Geometry: final body of the model. Coordinates: model frame, mm. A direction names the side the tool comes from. Round coordinates to 2 decimals unless told otherwise and drop trailing zeros. Write each loop counter-clockwise with the first axis right and the second up, starting at its lowest first coordinate (ties: lowest second). Pieces come first, ordered by that corner, then holes. Notation, with made-up numbers: (20, 30.5) - (72, 30.5) arc R24 ccw to (72, 60.5) - close; hole circle Ø3 at (70.5, -29.75). An arc over 180 degrees is marked (long way). Use a Markdown table: item, result. Add a question column.
```python
from build123d import *

# Parameters (mm, degrees)
ESQUISSE1_R             = 12
ESQUISSE1_R_2           = 1.5
ESQUISSE1_R_3           = 3
BOSS_EXTRU_1_DEPTH      = 2
BOSS_EXTRU_2_DEPTH      = 5
ESQUISSE3_R             = 1.25
ENL_V_MAT_EXTRU_1_DEPTH = 20.723082923


with BuildPart() as part:
    # Esquisse1 → Boss.-Extru.1 (new body)
    with BuildSketch(Plane.XY):
        Circle(ESQUISSE1_R)
        with Locations((-6.75, 0)):
            Circle(ESQUISSE1_R_2, mode=Mode.SUBTRACT)
        with Locations((6.75, 0)):
            Circle(ESQUISSE1_R_2, mode=Mode.SUBTRACT)
        Circle(ESQUISSE1_R_3, mode=Mode.SUBTRACT)
    extrude(amount=BOSS_EXTRU_1_DEPTH)

    # Esquisse2 → Boss.-Extru.2 (add)
    with BuildSketch(Plane.XY.offset(2)):
        with BuildLine():
            Line((-2, -2.236067977), (-2, -9))
            Line((-2, -9), (5, -9))
            Line((5, -9), (5, 9))
            Line((5, 9), (-2, 9))
            Line((-2, 9), (-2, 2.236067977))
            ThreePointArc((-2, 2.236067977), (3, 0), (-2, -2.236067977))
        make_face()
    extrude(amount=BOSS_EXTRU_2_DEPTH)

    # Esquisse3 → Enlèv. mat.-Extru.1 (cut, through all)
    with BuildSketch(Plane.ZY.offset(2)):
        with Locations(Location((4.5, 5.586067977, 0), (0, 0, 270))):
            Circle(ESQUISSE3_R)
        with Locations(Location((4.5, -5.586067977, 0), (0, 0, 270))):
            Circle(ESQUISSE3_R)
    extrude(amount=-ENL_V_MAT_EXTRU_1_DEPTH, mode=Mode.SUBTRACT)


solid = part.part
```
1) Section B-B, the plane z = 4.5. Return the cut outline in (x, y).
2) Set-up query: faces 1 (the flat face through (1, -9, 4)), 2 (the flat face through (-2, 6, 6)), 3 (the flat face through (2, 9, 4)), 4 (the flat face through (2.5, -2.5, 0)). Return all of +Z, -Z, +X, -X, +Y, -Y with unobstructed straight access to the full face (end or side cutting, diameter ignored); none if empty.
3) Material intervals for L1, parallel to Y at x = 2.75, z = 3.5; L2, parallel to Z at x = 8.5, y = 2.5; L3, parallel to X at y = 4.75, z = 2.25, sorted ascending. Write a range as from..to.
4) Draft query along X for faces 5 (the cylindrical face through (1.45, 5.01, 3.39)), 6 (the cylindrical face through (-8.25, 0.07, 0.99)), 7 (the flat face through (5, 0, 4)), 8 (the flat face through (-2, -5, 6)). Return one class per face: released by +X, released by -X, zero draft, split by the parting line, or undercut.
5) Section C-C, the plane x = 0. Return the cut outline in (y, z), then the cut area to 3 significant figures.
6) Section A-A, the plane y = 0. Return the cut outline in (x, z), then the cut area to 3 significant figures.
7) Section D-D, the plane x = 6.75. Return the cut outline in (y, z).
8) Pin query (flat end, axial travel): P1, Ø3, axis at x = 5, z = 5, coming from the +Y side; P2, Ø3, axis at x = -6.5, y = 5.5, coming from the +Z side; P3, Ø1.5, axis at x = 1, z = 3.5, coming from the -Y side. Return the tip coordinate at first contact, or that it passes through.
Output values:
| question | item | result |
|---|---|---|
| 1 | outline | (-2, -9) - (5, -9) - (5, -6.84) - (-2, -6.84) - close; (-2, -4.34) - (5, -4.34) - (5, 4.34) - (-2, 4.34) - (-2, 2.24) arc R3 cw (long way) to (-2, -2.24) - close; (-2, 6.84) - (5, 6.84) - (5, 9) - (-2, 9) - close |
| 2 | face 1 | +Z, +X, -X, -Y |
| 2 | face 2 | +Z, -X, +Y, -Y |
| 2 | face 3 | +Z, +X, -X, +Y |
| 2 | face 4 | -Z, +X, -X, +Y, -Y |
| 3 | L1 | y = -9..-6.34, -4.84..-1.2, 1.2..4.84, 6.34..9 |
| 3 | L2 | z = 0..2 |
| 3 | L3 | x = -2..5 |
| 4 | face 5 | zero draft |
| 4 | face 6 | undercut |
| 4 | face 7 | released by +X |
| 4 | face 8 | released by -X |
| 5 | outline | (-12, 0) - (-3, 0) - (-3, 7) - (-9, 7) - (-9, 2) - (-12, 2) - close; (3, 0) - (12, 0) - (12, 2) - (9, 2) - (9, 7) - (3, 7) - close; hole circle Ø2.5 at (-5.59, 4.5); hole circle Ø2.5 at (5.59, 4.5) |
| 5 | area | 86.2 mm^2 |
| 6 | outline | (-12, 0) - (-8.25, 0) - (-8.25, 2) - (-12, 2) - close; (-5.25, 0) - (-3, 0) - (-3, 2) - (-5.25, 2) - close; (3, 0) - (5.25, 0) - (5.25, 2) - (5, 2) - (5, 7) - (3, 7) - close; (8.25, 0) - (12, 0) - (12, 2) - (8.25, 2) - close |
| 6 | area | 34.0 mm^2 |
| 7 | outline | (-9.92, 0) - (-1.5, 0) - (-1.5, 2) - (-9.92, 2) - close; (1.5, 0) - (9.92, 0) - (9.92, 2) - (1.5, 2) - close |
| 8 | P1 | stops at y = 9 |
| 8 | P2 | stops at z = 2 |
| 8 | P3 | stops at y = -9 |
